The listing builds one solid part. Answer for the finished solid, in the listing's coordinates (mm). A direction names the side the tool comes from. Coordinates: 2 decimals unless noted, no trailing zeros. Loops run counter-clockwise (first coordinate to the right, second up) from the corner with the lowest first, then second, coordinate; pieces in that order, holes last. Notation, with made-up numbers: M 3.25,55.25 L 59.25,55.25 A20 cw 59.25,80.25 Z; hole C -37.75,78.5 d6. An arc over 180 degrees is marked long. Return JSON: item names as keys, results as strings. Group by question number.
1. Section A-A (y = 26.5) is taken. Write down the section's boundary in (x, z), then the cut area to 3 significant figures.
2. The mould has two halves that part along X. Classify faces 6 (the face through (-31.27, 43.84, -25.46)), 7 (the face through (49.2, 48.6, 47)), 8 (the face through (-35.995, 45.324, 24.7)), 9 (the face through (-1, 49, -48.578)): pulls with the +X half, pulls with the -X half, needs draft (parallel to the pull), parting line crosses it, or undercut.
3. Section C-C (y = 37) is taken. Write down the section's boundary in (x, z).
4. Given P1, Ø17.5, axis at y = 44, z = 13, coming from the -X side; P2, Ø7, axis at x = 48, y = 44.5, coming from the -Z side; P3, Ø3, axis at x = -21.5, y = 14.5, coming from the -Z side; P4, Ø12.5, axis at y = 49.5, z = 13, coming from the +X side, each flat-ended and moving along its own axis, determine where each tip first touches the part or whether it passes through.
5. Straight lines are drawn through the part: L1, parallel to Z at x = 43, y = 45.72; L2, parallel to X at y = 35.5, z = 39.5; L3, parallel to Y at x = 38.1, z = -44.5. For each, find the intervals that lie inside material, in ascending order. Write a range as from..to.
6. Section B-B (x = 0) is taken. Write down the section's boundary in (y, z) (1 decimal).
7. Which of the six approach directions +Z, -Z, +X, -X, +Y, -Y give full straight-line access (tool end or side, diameter ignored) to faces 1 (the face through (-19.05, 37, 43)), 2 (the face through (36.235, 58.217, 28.457)), 3 (the face through (-44.45, 47, -5)), 4 (the face through (48, 44, 37.148)), 5 (the face through (-30.659, 37.842, 38.768))?
```python
from build123d import *

# Parameters (mm, degrees)
SKETCH1_W                            = 101.6
SKETCH1_H                            = 97.155
BOSS_EXTRUDE1_DEPTH                  = 58.42
SKETCH2_W                            = 21.59
SKETCH2_H                            = 39.37
CUT_EXTRUDE1_DEPTH                   = 125.22813862
SKETCH3_R                            = 40.513
CUT_EXTRUDE2_DEPTH                   = 92.396443619
CUT_EXTRUDE3_START                   = -39.37
CUT_EXTRUDE3_DEPTH                   = 39.37
CUT_EXTRUDE4_REACH                   = 126.228
CUT_EXTRUDE4_END_RADIUS              = 40.513
SKETCH5_W                            = 38.1
SKETCH5_H                            = 48.895
FILLET1_R                            = 6.35
FILLET2_R                            = 5.08
CHAMFER1_SIZE                        = 3.175
CUT_EXTRUDE5_DEPTH                   = 6.35
TAP_DRILL_FOR_1_4_28_TAP1_AT_2_COUNT = 2
TAP_DRILL_FOR_1_4_28_TAP1_AT_2_PITCH = 44.45
TAP_DRILL_FOR_1_4_28_TAP2_D          = 5.4102
TAP_DRILL_FOR_1_4_28_TAP2_DEPTH      = 9.804611939
TAP_DRILL_FOR_1_4_28_TAP2_TIP        = 1.625388061
SKETCH12_R                           = 5.715
CUT_EXTRUDE6_DEPTH                   = 12.7
SKETCH13_R                           = 40.513
CUT_EXTRUDE7_DEPTH                   = 3.81
CHAMFER2_SIZE                        = 0.4


with BuildPart() as part:
    # Sketch1 → Boss-Extrude1 (new body)
    with BuildSketch(Plane(origin=(0, 0, 0), x_dir=(1, 0, 0), z_dir=(0, 1, 0))):
        Rectangle(SKETCH1_W, SKETCH1_H)
    extrude(amount=BOSS_EXTRUDE1_DEPTH)

    # Sketch2 → Cut-Extrude1 (cut, through all)
    with BuildSketch(Plane.XY.offset(48.5775)):
        with Locations((-40.005, 19.685)):
            Rectangle(SKETCH2_W, SKETCH2_H)
        with Locations((40.005, 19.685)):
            Rectangle(SKETCH2_W, SKETCH2_H)
    extrude(amount=-CUT_EXTRUDE1_DEPTH, mode=Mode.SUBTRACT)

    # Sketch3 → Cut-Extrude2 (cut, through all)
    with BuildSketch(Plane(origin=(0, 58.42, 0), x_dir=(1, 0, 0), z_dir=(0, 1, 0))):
        with Locations(Location((0, -2.2225, 0), (0, 0, 270))):
            Circle(SKETCH3_R)
    extrude(amount=-CUT_EXTRUDE2_DEPTH, mode=Mode.SUBTRACT)

    # Sketch4 → Cut-Extrude3 (cut)
    with BuildSketch(Plane.XZ.offset(CUT_EXTRUDE3_START)):
        with BuildLine():
            Line((-29.21, -25.850246018), (-29.21, -48.5775))
            Line((-29.21, -48.5775), (29.21, -48.5775))
            Line((29.21, -48.5775), (29.21, -25.850246018))
            ThreePointArc((29.21, -25.850246018), (0, -38.2905), (-29.21, -25.850246018))
        make_face()
    extrude(amount=CUT_EXTRUDE3_DEPTH, mode=Mode.SUBTRACT)

    # Cut-Extrude4: up to this cylinder (the profile starts outside it)
    cut_extrude4_end = Plane(origin=(0, 33.9725, 2.2225), z_dir=(0, 1, 0)) * Cylinder(CUT_EXTRUDE4_END_RADIUS, 334.482, mode=Mode.PRIVATE)
    # Sketch5 → Cut-Extrude4 (cut, up to the surface)
    with BuildSketch(Plane.XY.offset(48.5775), mode=Mode.PRIVATE) as cut_extrude4_sk1:
        with Locations((0, 33.9725)):
            Rectangle(SKETCH5_W, SKETCH5_H)
    cut_extrude4_tool1 = extrude(cut_extrude4_sk1.sketch, amount=-CUT_EXTRUDE4_REACH, mode=Mode.PRIVATE) - cut_extrude4_end
    add(cut_extrude4_tool1.solids().sort_by_distance((0, 33.9725, 48.5775))[0], mode=Mode.SUBTRACT)

    # Fillet1
    fillet1_edges = [part.edges().sort_by_distance(p)[0] for p in [
        (-29.21, 0, 39.436373009),
        (29.21, 0, 39.436373009),
        (-19.05, 9.525, 43.277364662),
        (19.05, 9.525, 43.277364662),
    ]]
    fillet(fillet1_edges, radius=FILLET1_R)

    # Fillet2
    fillet2_edges = [part.edges().sort_by_distance(p)[0] for p in [
        (-29.21, 39.37, 39.436373009),
        (29.21, 39.37, 39.436373009),
    ]]
    fillet(fillet2_edges, radius=FILLET2_R)

    # Chamfer1
    chamfer1_edges = [part.edges().sort_by_distance(p)[0] for p in [
        (50.8, 48.895, 48.5775),
        (-50.8, 48.895, 48.5775),
    ]]
    chamfer(chamfer1_edges, length=CHAMFER1_SIZE)

    # Sketch6 → Cut-Extrude5 (cut)
    with BuildSketch(Plane.ZY.offset(50.8)):
        with BuildLine():
            Line((-48.5775, 55.245), (30.7975, 55.245))
            ThreePointArc((30.7975, 55.245), (35.287628061, 53.385128061), (37.1475, 48.895))
            Line((37.1475, 48.895), (37.1475, 39.37))
            Line((37.1475, 39.37), (-48.5775, 39.37))
            Line((-48.5775, 39.37), (-48.5775, 55.245))
        make_face()
    cut_extrude5 = extrude(amount=-CUT_EXTRUDE5_DEPTH, mode=Mode.SUBTRACT)

    # Sketch8 → Tap Drill for 1/4-28 Tap1 (revolve, cut)
    with BuildSketch(Plane(origin=(-44.45, 45.72, -20.0025), x_dir=(0, 0, 1), z_dir=(0, 1, 0))):
        Polygon((0, 0), (0, 8.737388061), (2.7051, 7.112), (2.7051, 0), align=None)
    tap_drill_for_1_4_28_tap1 = revolve(axis=Axis((-50.8, 45.72, -20.0025), (1, 0, 0)), mode=Mode.SUBTRACT)

    # Tap Drill for 1/4-28 Tap1 at 2: Tap Drill for 1/4-28 Tap1 ×2
    with Locations(*[(0, 0, i * TAP_DRILL_FOR_1_4_28_TAP1_AT_2_PITCH) for i in range(1, TAP_DRILL_FOR_1_4_28_TAP1_AT_2_COUNT)]):
        add(tap_drill_for_1_4_28_tap1, mode=Mode.SUBTRACT)

    # Tap Drill for 1/4-28 Tap2
    with Locations(Plane(origin=(38.1, 48.895, -48.5775), x_dir=(-1, 0, 0), z_dir=(0, 0, -1))):
        with Locations((0, 0), (76.2, 0)):
            Hole(TAP_DRILL_FOR_1_4_28_TAP2_D / 2, depth=TAP_DRILL_FOR_1_4_28_TAP2_DEPTH)
            with Locations((0, 0, -(TAP_DRILL_FOR_1_4_28_TAP2_DEPTH + TAP_DRILL_FOR_1_4_28_TAP2_TIP / 2))):  # 118° drill point
                Cone(0, TAP_DRILL_FOR_1_4_28_TAP2_D / 2, TAP_DRILL_FOR_1_4_28_TAP2_TIP, mode=Mode.SUBTRACT)

    # Sketch12 → Cut-Extrude6 (cut)
    with BuildSketch(Plane(origin=(0, 58.42, 0), x_dir=(1, 0, 0), z_dir=(0, 1, 0))):
        with Locations((-32.2961, 31.4452)):
            Circle(SKETCH12_R)
        with BuildLine():
            ThreePointArc((-33.992836913, 19.818148984), (-20.14878741, 32.924755012), (-1.84310515, 38.248553018))
            Line((-1.84310515, 38.248553018), (-32.499537967, 37.156577942))
            ThreePointArc((-32.499537967, 37.156577942), (-28.327562674, 35.55761249), (-26.5811, 31.4452))
            ThreePointArc((-26.5811, 31.4452), (-31.264433085, 25.824089044), (-37.638628741, 29.41576371))
            Line((-37.638628741, 29.41576371), (-33.992836913, 19.818148984))
        make_face()
        with BuildLine():
            Line((32.499537967, 37.156577942), (1.84310515, 38.248553018))
            ThreePointArc((1.84310515, 38.248553018), (20.14878741, 32.924755012), (33.992836913, 19.818148984))
            Line((33.992836913, 19.818148984), (37.638628741, 29.41576371))
            ThreePointArc((37.638628741, 29.41576371), (27.534851432, 28.284229093), (32.499537967, 37.156577942))
        make_face()
        with Locations((32.2961, 31.4452)):
            Circle(SKETCH12_R)
        with Locations((32.84347, -35.17392)):
            Circle(SKETCH12_R)
        with BuildLine():
            Line((38.023019003, -32.758656634), (34.032742491, -24.20148104))
            ThreePointArc((34.032742491, -24.20148104), (27.420561588, -32.045577829), (19.05, -37.977229324))
            Line((19.05, -37.977229324), (19.05, -41.349640271))
            Line((19.05, -41.349640271), (33.032951844, -40.885777984))
            ThreePointArc((33.032951844, -40.885777984), (27.973239162, -32.183589486), (38.023019003, -32.758656634))
        make_face()
        with BuildLine():
            ThreePointArc((-19.05, -37.977229324), (-27.420561588, -32.045577829), (-34.032742491, -24.20148104))
            Line((-34.032742491, -24.20148104), (-38.023019003, -32.758656634))
            ThreePointArc((-38.023019003, -32.758656634), (-31.606517606, -29.594388319), (-27.12847, -35.17392))
            ThreePointArc((-27.12847, -35.17392), (-28.869911377, -39.281480939), (-33.032951844, -40.885777984))
            Line((-33.032951844, -40.885777984), (-19.05, -41.349640271))
            Line((-19.05, -41.349640271), (-19.05, -37.977229324))
        make_face()
        with Locations((-32.84347, -35.17392)):
            Circle(SKETCH12_R)
    extrude(amount=-CUT_EXTRUDE6_DEPTH, mode=Mode.SUBTRACT)

    # Sketch13 → Cut-Extrude7 (cut)
    with BuildSketch(Plane(origin=(0, 45.72, 0), x_dir=(1, 0, 0), z_dir=(0, 1, 0))):
        with BuildLine():
            Line((-27.928285617, 34.477511324), (-30.468285617, 35.038851324))
            ThreePointArc((-30.468285617, 35.038851324), (-36.146291324, 31.416274383), (-32.523714383, 25.738268676))
            Line((-32.523714383, 25.738268676), (-29.983714383, 25.176928676))
            ThreePointArc((-29.983714383, 25.176928676), (-29.924483296, 25.164233151), (-29.865095524, 25.152292024))
            ThreePointArc((-29.865095524, 25.152292024), (-27.159369973, 27.838634238), (-24.213087874, 30.258718336))
            ThreePointArc((-24.213087874, 30.258718336), (-25.381844695, 32.974730144), (-27.928285617, 34.477511324))
        make_face()
        with Locations(Location((0, -2.2225, 0), (0, 0, 288.269054449))):
            Circle(SKETCH13_R)
        with BuildLine():
            ThreePointArc((-27.62071326, -36.63561929), (-26.67134071, -29.96767326), (-33.33928674, -29.01830071))
            Line((-33.33928674, -29.01830071), (-35.07156674, -30.31878071))
            ThreePointArc((-35.07156674, -30.31878071), (-36.02093929, -36.98672674), (-29.35299326, -37.93609929))
            Line((-29.35299326, -37.93609929), (-27.62071326, -36.63561929))
        make_face()
    cut_extrude7 = extrude(amount=-CUT_EXTRUDE7_DEPTH, mode=Mode.SUBTRACT)

    # Mirror1: Cut-Extrude5, Tap Drill for 1/4-28 Tap1, Cut-Extrude7 across plane
    add(cut_extrude5.mirror(Plane(origin=(0, 0, 0), x_dir=(0, 0, 1), z_dir=(1, 0, 0))), mode=Mode.SUBTRACT)
    add(tap_drill_for_1_4_28_tap1.mirror(Plane(origin=(0, 0, 0), x_dir=(0, 0, 1), z_dir=(1, 0, 0))), mode=Mode.SUBTRACT)
    add(cut_extrude7.mirror(Plane(origin=(0, 0, 0), x_dir=(0, 0, 1), z_dir=(1, 0, 0))), mode=Mode.SUBTRACT)

    # Mirror1 copy 1 sketch → Mirror1 copy 1 (revolve, cut)
    with BuildSketch(Plane(origin=(44.45, 45.72, 24.4475), x_dir=(0, 0, 1), z_dir=(0, 1, 0))):
        Polygon((0, 0), (0, -8.737388061), (2.7051, -7.112), (2.7051, 0), align=None)
    revolve(axis=Axis((50.8, 45.72, 24.4475), (1, 0, 0)), mode=Mode.SUBTRACT)

    # Chamfer2
    chamfer2_edges = [part.edges().sort_by_distance(p)[0] for p in [
        (50.8, 58.42, -1.5875),
        (-33.3375, 58.42, 48.5775),
        (-49.2125, 58.42, 46.99),
        (49.2125, 58.42, 46.99),
        (0, 58.42, -48.5775),
        (19.05, 58.42, 44.963570135),
        (-19.05, 58.42, 44.963570135),
        (40.512983353, 58.42, 2.185773339),
        (0, 58.42, -38.2905),
        (-40.512983353, 58.42, 2.185773339),
        (-36.027880747, 58.42, 28.480068837),
        (-37.713700838, 58.42, 38.164250514),
        (-26.041475922, 58.42, 41.117709128),
        (37.713700838, 58.42, 38.164250514),
        (36.027880747, 58.42, 28.480068837),
        (26.041475922, 58.42, 41.117709128),
        (17.171321559, 58.42, -37.70256548),
        (35.815732827, 58.42, -24.616956347),
        (37.057348568, 58.42, -34.606170907),
        (-35.815732827, 58.42, -24.616956347),
        (-37.057348568, 58.42, -34.606170907),
        (-17.171321559, 58.42, -37.70256548),
        (-50.8, 58.42, -1.5875),
        (33.3375, 58.42, 48.5775),
    ]]
    chamfer(chamfer2_edges, length=CHAMFER2_SIZE)


solid = part.part
```
Worked out:
{
 "1": {"outline": "M -29.21,30.3 A40.51 cw -19.05,37.98 L -19.05,48.58 L -29.21,48.58 Z; M 19.05,37.98 A40.51 cw 29.21,30.3 L 29.21,48.58 L 19.05,48.58 Z", "area": "285 mm^2"},
 "2": {"face 6": "undercut", "face 7": "pulls with the +X half", "face 8": "pulls with the -X half", "face 9": "needs draft"},
 "3": {"outline": "M -29.99,29.46 A40.51 cw -19.05,37.98 L -19.05,48.58 L -29.99,48.58 Z; M 19.05,37.98 A40.51 cw 29.99,29.46 L 29.99,48.58 L 19.05,48.58 Z"},
 "4": {"P1": "x = -44.45", "P2": "z = 37.15", "P3": "z = 35.57", "P4": "x = 50.8"},
 "5": {"L1": "-48.58..-22.71, -17.3..21.74, 27.15..48.58", "L2": "-29.36..-19.05, 19.05..29.36", "L3": "39.37..46.19, 51.6..58.42"},
 "6": {"outline": "M 0,42.7 L 9.5,42.7 L 9.5,48.6 L 0,48.6 Z; M 39.4,-48.6 L 58,-48.6 L 58.4,-48.2 L 58.4,-38.7 L 58,-38.3 L 39.4,-38.3 Z"},
 "7": {"face 1": "+Z, +Y", "face 2": "+Y", "face 3": "-Z, -X, -Y", "face 4": "-Z, +X, -Y", "face 5": "+Z, -Z, -X, -Y"}
}
